For this review, take the finished solid that the model builds, in its own axes (mm). Face numbers are marked on the shaded views. A direction names the side the tool comes from. Give positions to 0.01 mm unless a question says otherwise; leave off trailing zeros. Loops run counter-clockwise (first coordinate to the right, second up) from the corner with the lowest first, then second, coordinate; pieces in that order, holes last. Notation, with made-up numbers: M 54.5,15.25 L 88.5,15.25 A12 cw 88.5,34.25 Z; hole C 60,76 d11. An arc over 180 degrees is marked long. Use CSV: the item, a comma, the result in double quotes. Start each with the question number.
1. Tool access review of the marked faces 1, 2, 3 and 4: name each direction out of +Z, -Z, +X, -X, +Y, -Y from which nothing blocks a thin tool from reaching the whole face with its end or side.
2. Take a section at B-B, the plane z = 1. Write out the cut boundary in (x, y).
3. Take a section at D-D, the plane y = -9.5. Write out the cut boundary in (x, z).
4. The part is to be moulded in two halves that separate along X. For the marked faces 5, 6 and 7, say which applies: pulls with the +X half, pulls with the -X half, needs draft (parallel to the pull), parting line crosses it, or undercut.
5. Insertion check: P1, Ø2, axis at y = 0.5, z = -6.5, coming from the +X side; P2, Ø20, axis at x = 89, y = 29, coming from the +Z side; P3, Ø20, axis at x = -83, y = 25, coming from the +Z side. Each pin has a flat end and moves straight along its axis. Give the tip position at first contact, or say it passes through.
6. To check wall thickness, follow line 1 (X direction, y = -30.5, z = 7); line 2 (X direction, y = 52, z = -13.5); line 3 (Z direction, x = 54, y = -49). State the ranges of each line that lie inside material, in increasing order. Write a range as [from, to].
7. Take a section at C-C, the plane x = 85. Write out the cut boundary in (y, z), and give its area (3 significant figures).
8. Take a section at A-A, the plane y = 39. Write out the cut boundary in (x, z), and give its area (3 significant figures).
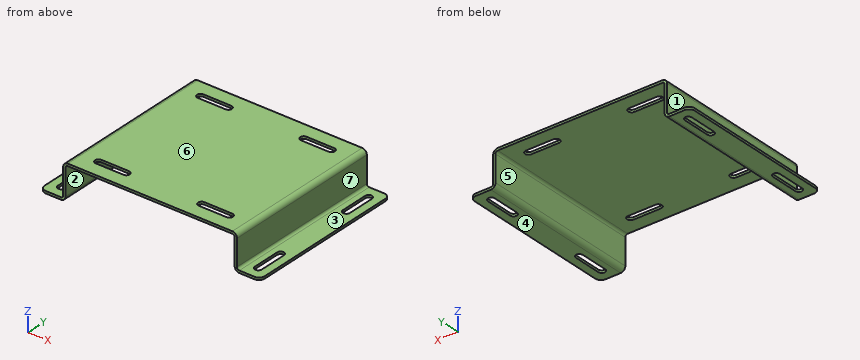
from build123d import *

# Parameters (mm, degrees)
F1_DEPTH = 70
F2_R     = 2
F3_R     = 4
F5_DEPTH = 25
F6_R     = 5
F8_DEPTH = 25


with BuildPart() as f1:
    # F0 (on Front) → F1 (new body, symmetric)
    with BuildSketch(Plane.XZ):
        Polygon((75, 15.3), (-75, 15.3), (-75, -13.3), (-95, -13.3), (-95, -15.3), (-75, -15.3), (-73, -15.3), (-73, -13.3), (-73, 13.3), (73, 13.3), (73, -13.3), (73, -15.3), (75, -15.3), (95, -15.3), (95, -13.3), (75, -13.3), align=None)
    extrude(amount=F1_DEPTH, both=True)

    # F2
    f2_edges = [f1.edges().sort_by_distance(p)[0] for p in [
        (-73, 0, 13.3),
        (73, 0, 13.3),
        (75, 0, -13.3),
        (-75, 0, -13.3),
    ]]
    fillet(f2_edges, radius=F2_R)

    # F3
    f3_edges = [f1.edges().sort_by_distance(p)[0] for p in [
        (-75, 0, 15.3),
        (-73, 0, -15.3),
        (73, 0, -15.3),
        (75, 0, 15.3),
    ]]
    fillet(f3_edges, radius=F3_R)

    # F4 (on face) → F5 (cut)
    with BuildSketch(Plane.XY.offset(-13.3)):
        with BuildLine():
            Line((-82, 35.5), (-82, 59.5))
            ThreePointArc((-82, 59.5), (-85, 62.5), (-88, 59.5))
            Line((-88, 59.5), (-88, 35.5))
            ThreePointArc((-88, 35.5), (-85, 32.5), (-82, 35.5))
        make_face()
        with BuildLine():
            Line((-88, -35.5), (-88, -59.5))
            ThreePointArc((-88, -59.5), (-85, -62.5), (-82, -59.5))
            Line((-82, -59.5), (-82, -35.5))
            ThreePointArc((-82, -35.5), (-85, -32.5), (-88, -35.5))
        make_face()
        with BuildLine():
            Line((82, -35.5), (82, -59.5))
            ThreePointArc((82, -59.5), (85, -62.5), (88, -59.5))
            Line((88, -59.5), (88, -35.5))
            ThreePointArc((88, -35.5), (85, -32.5), (82, -35.5))
        make_face()
        with BuildLine():
            ThreePointArc((88, 59.5), (85, 62.5), (82, 59.5))
            Line((82, 59.5), (82, 35.5))
            ThreePointArc((82, 35.5), (85, 32.5), (88, 35.5))
            Line((88, 35.5), (88, 59.5))
        make_face()
    extrude(amount=-F5_DEPTH, mode=Mode.SUBTRACT)

    # F6
    f6_edges = [f1.edges().sort_by_distance(p)[0] for p in [
        (-95, 70, -14.3),
        (95, 70, -14.3),
        (-95, -70, -14.3),
        (95, -70, -14.3),
    ]]
    fillet(f6_edges, radius=F6_R)

    # F7 (on face) → F8 (cut)
    with BuildSketch(Plane.XY.offset(15.3)):
        with BuildLine():
            Line((-56.5, 52), (-32.5, 52))
            ThreePointArc((-32.5, 52), (-29.5, 55), (-32.5, 58))
            Line((-32.5, 58), (-56.5, 58))
            ThreePointArc((-56.5, 58), (-59.5, 55), (-56.5, 52))
        make_face()
        with BuildLine():
            ThreePointArc((32.5, 58), (29.5, 55), (32.5, 52))
            Line((32.5, 52), (56.5, 52))
            ThreePointArc((56.5, 52), (59.5, 55), (56.5, 58))
            Line((56.5, 58), (32.5, 58))
        make_face()
        with BuildLine():
            Line((32.5, -58), (56.5, -58))
            ThreePointArc((56.5, -58), (59.5, -55), (56.5, -52))
            Line((56.5, -52), (32.5, -52))
            ThreePointArc((32.5, -52), (29.5, -55), (32.5, -58))
        make_face()
        with BuildLine():
            ThreePointArc((-32.5, -58), (-29.5, -55), (-32.5, -52))
            Line((-32.5, -52), (-56.5, -52))
            ThreePointArc((-56.5, -52), (-59.5, -55), (-56.5, -58))
            Line((-56.5, -58), (-32.5, -58))
        make_face()
    extrude(amount=-F8_DEPTH, mode=Mode.SUBTRACT)


solid = f1.part
Result set:
1,face 1,"+Z, -X, +Y, -Y"
1,face 2,"-Z, +Y, -Y"
1,face 3,"+Z, +X, +Y, -Y"
1,face 4,"-Z, +X, -X, +Y, -Y"
2,outline,"M -75,-70 L -73,-70 L -73,70 L -75,70 Z; M 73,-70 L 75,-70 L 75,70 L 73,70 Z"
3,outline,"M -95,-15.3 L -77,-15.3 A4 ccw -73,-11.3 L -73,11.3 A2 cw -71,13.3 L 71,13.3 A2 cw 73,11.3 L 73,-11.3 A4 ccw 77,-15.3 L 95,-15.3 L 95,-13.3 L 77,-13.3 A2 cw 75,-11.3 L 75,11.3 A4 ccw 71,15.3 L -71,15.3 A4 ccw -75,11.3 L -75,-11.3 A2 cw -77,-13.3 L -95,-13.3 Z"
4,face 5,"undercut"
4,face 6,"needs draft"
4,face 7,"pulls with the +X half"
5,P1,"x = 75"
5,P2,"z = -13.3"
5,P3,"z = 14.76"
6,line 1,"[-75, -73], [73, 75]"
6,line 2,"[-95, -88], [-82, -73.66], [73.66, 82], [88, 95]"
6,line 3,"[13.3, 15.3]"
7,outline,"M -70,-15.3 L -62.5,-15.3 L -62.5,-13.3 L -70,-13.3 Z; M -32.5,-15.3 L 32.5,-15.3 L 32.5,-13.3 L -32.5,-13.3 Z; M 62.5,-15.3 L 70,-15.3 L 70,-13.3 L 62.5,-13.3 Z"
7,area,"160 mm2"
8,outline,"M -95,-15.3 L -88,-15.3 L -88,-13.3 L -95,-13.3 Z; M -82,-15.3 L -77,-15.3 A4 ccw -73,-11.3 L -73,11.3 A2 cw -71,13.3 L 71,13.3 A2 cw 73,11.3 L 73,-11.3 A4 ccw 77,-15.3 L 82,-15.3 L 82,-13.3 L 77,-13.3 A2 cw 75,-11.3 L 75,11.3 A4 ccw 71,15.3 L -71,15.3 A4 ccw -75,11.3 L -75,-11.3 A2 cw -77,-13.3 L -82,-13.3 Z; M 88,-15.3 L 95,-15.3 L 95,-13.3 L 88,-13.3 Z"
8,area,"460 mm2"
